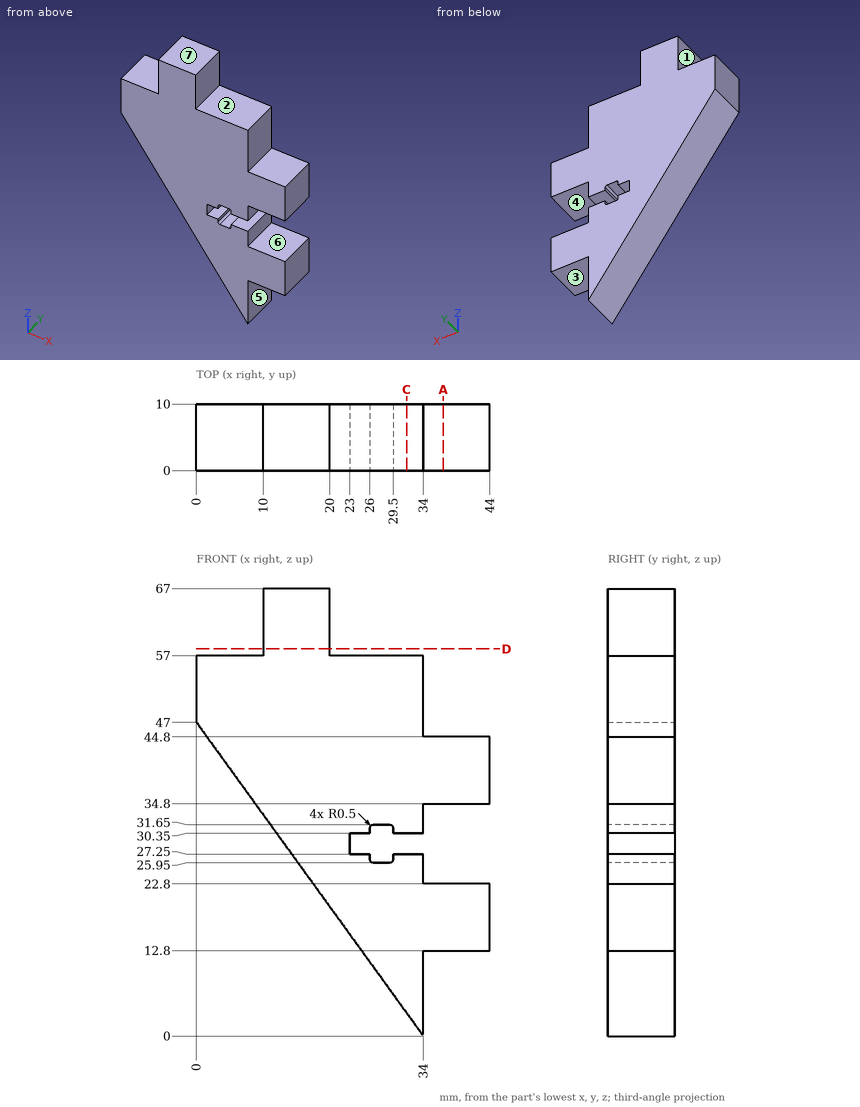
Study the drawing (mm; zero at the part's minimum x, y, z) and answer. A direction names the side the tool comes from. Give positions to 0.01 mm unless a question says otherwise; leave off trailing zeros. Loops run counter-clockwise (first coordinate to the right, second up) from the corner with the lowest first, then second, coordinate; pieces in that order, holes last. Notation, with made-up numbers: M 22.5,82 L 35.5,82 A18 ccw 35.5,113 Z; hole C 3.25,-38.75 d2. An arc over 180 degrees is marked long. One line per item, written item: value. Start each with the question number.
1. Find section C-C (x = 31.5). Give the vertices of the cut face in (y, z), and give its area (3 significant figures).
2. Find the intervals of material crossed by probe 1 along X at (y, z) = (4.25, 51); probe 2 along X at (y, z) = (0.75, 60); probe 3 along X at (y, z) = (4.25, 27), in increasing order.
3. Which of the six approach directions +Z, -Z, +X, -X, +Y, -Y give full straight-line access (tool end or side, diameter ignored) to the marked faces 1, 2, 3 and 4?
4. Find section D-D (z = 58). Give the vertices of the cut face in (x, y), and give its area (3 significant figures).
5. Determine the mould class of the marked faces 5, 6 and 7 for opening direction Z: released by +Z, released by -Z, zero draft, split by the parting line, or undercut.
6. Each of these flat-tipped pins is pushed along its axis until it touches: P1, Ø3, axis at x = 28, y = 5, coming from the -Z side; P2, Ø5, axis at x = 38.5, y = 3.5, coming from the -Z side; P3, Ø4, axis at x = 23, y = 8.5, coming from the -Z side. Where does it stop, or does it pass through?
7. Find section A-A (x = 37). Give the vertices of the cut face in (y, z), and give its area (3 significant figures).
Reported:
1. outline: M 0,3.46 L 10,3.46 L 10,27.25 L 0,27.25 Z; M 0,30.35 L 10,30.35 L 10,57 L 0,57 Z
1. area: 504 mm²
2. probe 1: x = 0 to 34
2. probe 2: x = 10 to 20
2. probe 3: x = 14.47 to 26, 29.5 to 34
3. face 1: +Z, -X, +Y, -Y
3. face 2: +Z, +X, +Y, -Y
3. face 3: -Z, +X, +Y, -Y
3. face 4: +X, +Y, -Y
4. outline: M 10,0 L 20,0 L 20,10 L 10,10 Z
4. area: 100 mm²
5. face 5: zero draft
5. face 6: undercut
5. face 7: released by +Z
6. P1: stops at z = 6.22
6. P2: stops at z = 12.8
6. P3: stops at z = 12.44
7. outline: M 0,12.8 L 10,12.8 L 10,22.8 L 0,22.8 Z; M 0,34.8 L 10,34.8 L 10,44.8 L 0,44.8 Z
7. area: 200 mm²
